Source: CAD feature listing. Evaluate the final solid. Frame: model axes, mm. Round coordinates to 2 decimals unless told otherwise and drop trailing zeros. Write each loop counter-clockwise with the first axis right and the second up, starting at its lowest first coordinate (ties: lowest second). Pieces come first, ordered by that corner, then holes. Notation, with made-up numbers: M 44.5,37.25 L 84.5,37.25 A15 cw 84.5,42.25 Z; hole C -4.75,75.5 d8. An arc over 180 degrees is marked long. Use a Markdown table: item, result.
```python
from build123d import *

# Parameters (mm, degrees)
F1_DEPTH = 0.9
F2_R     = 0.2
F3_R     = 0.5


with BuildPart() as f1:
    # F0 (on Front) → F1 (new body)
    with BuildSketch(Plane.XZ):
        Polygon((-20, 3.115), (-20, 0), (-20, -3.115), (0, -3.115), (1.885, -5), (80, -5), (80, 0), (80, 5), (1.885, 5), (0, 3.115), align=None)
    extrude(amount=F1_DEPTH)

    # F2
    f2_edges = [f1.edges().sort_by_distance(p)[0] for p in [
        (-20, -0.45, -3.115),
        (-20, -0.45, 3.115),
    ]]
    fillet(f2_edges, radius=F2_R)

    # F3
    f3_edges = [f1.edges().sort_by_distance(p)[0] for p in [
        (80, -0.45, -5),
        (80, -0.45, 5),
    ]]
    fillet(f3_edges, radius=F3_R)


solid = f1.part
```
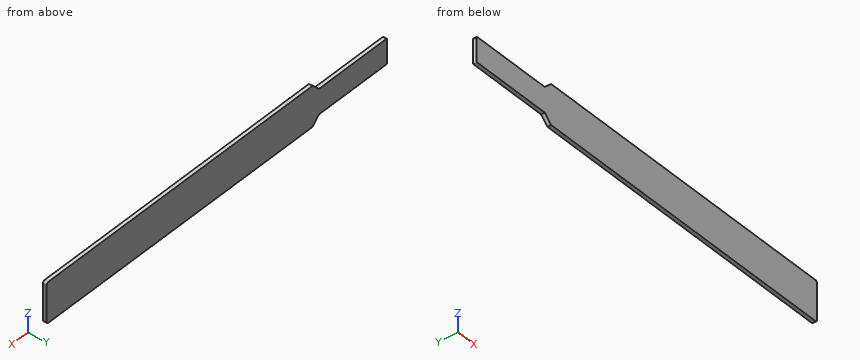
Q1. First-contact query: pin 1 Ø5 at (x, z) = (23.5, 4) entering from +Y. Flat tip, straight axial feed; report the tip coordinate or a pass-through.
Results are:
| item | result |
|---|---|
| pin 1 | y = 0 |
Q2. Section B-B on x = -13. Return loops of the section in (y, z) (3 decimals), plus the area to 3 significant figures.
Results are:
| item | result |
|---|---|
| outline | M -0.9,-3.115 L 0,-3.115 L 0,3.115 L -0.9,3.115 Z |
| area | 5.61 mm^2 |
Q3. Section A-A on y = -0.4. Return loops of the section in (x, z) (3 decimals), plus the area to 3 significant figures.
Results are:
| item | result |
|---|---|
| outline | M -20,-2.915 A0.2 ccw -19.8,-3.115 L 0,-3.115 L 1.885,-5 L 79.5,-5 A0.5 ccw 80,-4.5 L 80,4.5 A0.5 ccw 79.5,5 L 1.885,5 L 0,3.115 L -19.8,3.115 A0.2 ccw -20,2.915 Z |
| area | 921 mm^2 |
Q4. Line query: L1, parallel to Z at x = -8.5, y = -0.4 (3 decimals); L2, parallel to X at y = -0.3, z = 3.5 (3 decimals); L3, parallel to X at y = -0.7, z = 3. Output: solid intervals per line, ascending.
Results are:
| item | result |
|---|---|
| L1 | -3.115 to 3.115 |
| L2 | 0.385 to 80 |
| L3 | -19.98 to 80 |
